Answer from the drawing. Dimensions are ordinates in mm from the lowest x, y and z of the part. Round coordinates to 2 decimals unless told otherwise and drop trailing zeros. Loops run counter-clockwise (first coordinate to the right, second up) from the corner with the lowest first, then second, coordinate; pieces in that order, holes last. Notation, with made-up numbers: M -7,51.25 L -2,51.25 A9 cw -2,67.25 Z; hole C -10,25 d6. An arc over 180 degrees is marked long. Answer as CSV lines item,"result".
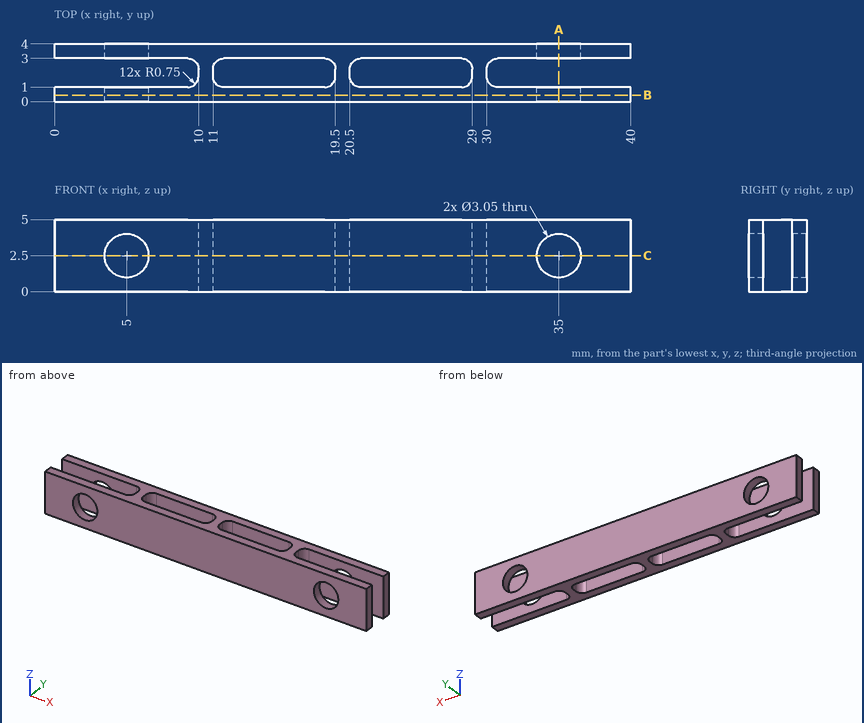
1) Each of these flat-tipped pins is pushed along its axis until it touches: P1, Ø1.8, axis at x = 5, z = 2.5, coming from the +Y side; P2, Ø2.5, axis at x = 25.5, z = 3.5, coming from the -Y side. Where does it stop, or does it pass through?
Evaluation:
P1,"passes through"
P2,"stops at y = 0"
2) Find section B-B, the plane y = 0.45. Give the vertices of the cut face in (x, z) (3 decimals).
Evaluation:
outline,"M 0,0 L 40,0 L 40,5 L 0,5 Z; hole C 5,2.5 d3.05; hole C 35,2.5 d3.05"
3) Find section A-A, the plane x = 35. Give the vertices of the cut face in (y, z) (3 decimals), then the cut area to 3 significant figures.
Evaluation:
outline,"M 0,0 L 1,0 L 1,0.975 L 0,0.975 Z; M 0,4.025 L 1,4.025 L 1,5 L 0,5 Z; M 3,0 L 4,0 L 4,0.975 L 3,0.975 Z; M 3,4.025 L 4,4.025 L 4,5 L 3,5 Z"
area,"3.90 mm^2"
4) Find section C-C, the plane z = 2.5. Count the separate pieces of the cut face and the enclosed holes in it, then the cut area to 3 significant figures.
Evaluation:
separate pieces,"5"
enclosed holes,"2"
area,"75.2 mm^2"
5) Straight lines are drawn through the part: line 1 (X direction, y = 0.7, z = 2.45); line 2 (X direction, y = 1.9, z = 3.75); line 3 (Y direction, x = 13, z = 2.4). For each, find the intervals that lie inside material, in ascending order.
Evaluation:
line 1,"x = 0 to 3.48, 6.52 to 33.48, 36.52 to 40"
line 2,"x = 10 to 11, 19.5 to 20.5, 29 to 30"
line 3,"y = 0 to 1, 3 to 4"
